```python
from build123d import *

# Parameters (mm, degrees)
F1_DEPTH = 25.4
F3_D     = 6.35
F3_DEPTH = 0.0254
F3_TIP   = 1.9077324654
F5_D     = 6.35


with BuildPart() as f1:
    # F0 (on Right) → F1 (new body)
    with BuildSketch(Plane.YZ):
        Polygon((19.0030846266, 19.1524188638), (12.6530846266, 19.1524188638), (12.6530846266, -6.2475811362), (-25.4469153734, -6.2475811362), (-25.4469153734, -12.5975811362), (19.0030846266, -12.5975811362), align=None)
    extrude(amount=F1_DEPTH)

    # F3
    with Locations(Plane(origin=(0, 19.0030846266, 0), x_dir=(-1, 0, 0), z_dir=(0, 1, 0))):
        with Locations((-12.7, 0.1024188638)):
            Hole(F3_D / 2, depth=F3_DEPTH)
            with Locations((0, 0, -(F3_DEPTH + F3_TIP / 2))):  # 118° drill point
                Cone(0, F3_D / 2, F3_TIP, mode=Mode.SUBTRACT)

    # F5 (through all)
    with Locations(Plane.XY.offset(-6.2475811362)):
        with Locations((12.7, -5.1269153734)):
            Hole(F5_D / 2)


solid = f1.part
```
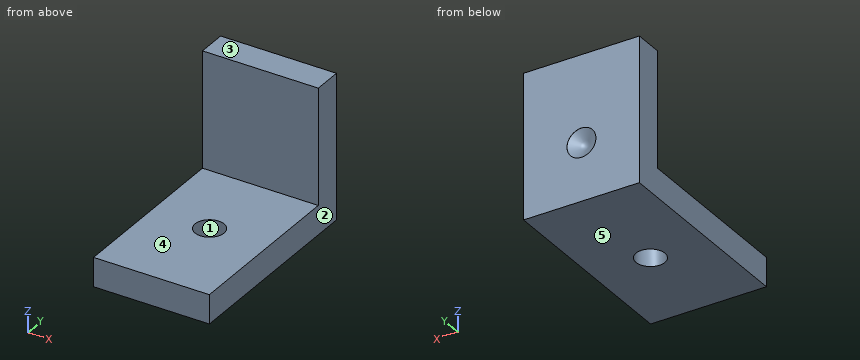
Geometry check sheet. Reference: the model listing, model coordinates, mm. Face numbers are marked on the shaded views. A direction names the side the tool comes from. Give positions to 0.01 mm unless a question says otherwise; leave off trailing zeros. Order: outer loops, then holes, each group sorted by start corner. A loop starts at its lowest first (then second) coordinate and runs counter-clockwise, first axis right, second up. Notation, with made-up numbers: (44, 48) -> (103, 48) arc R18 cw to (103, 77) -> close; hole circle Ø7 at (84, 48). An arc over 180 degrees is marked (long way). Write each question's results on one line, items separated by ' | '. Start each with the question number.
(1) Gauge pin test, flat ends, axial feed: P1, Ø12.5, axis at x = 16, z = 8.5, coming from the -Y side; P2, Ø8, axis at x = 19, y = -21, coming from the +Z side. Record the tip position at first contact, or that the pin passes through.
(2) Mould release check, pull along X, two halves, no side actions. Record for the marked faces 1, 2 and 3: pulls with the +X half, pulls with the -X half, needs draft (parallel to the pull), parting line crosses it, or undercut.
(3) Sectioned sample at A-A (z = 13.5). Enter the section's corners in (x, y).
(4) Scan lines: line 1 (Y direction, x = 12.7, z = -8); line 2 (Y direction, x = 1, z = 11); line 3 (Z direction, x = 16.25, y = -6.5). Record each from-to range of solid material in increasing order.
(5) Sectioned sample at C-C (y = -10). Enter the section's corners in (x, z).
(6) Sectioned sample at B-B (x = 17.25). Enter the section's corners in (y, z).
(7) Access from +Z, -Z, +X, -X, +Y, -Y to the whole of each face (thin tool, end or side, straight path). Record for the marked faces 4 and 5.
Answer below:
1) P1: y = 12.65 | P2: z = -6.25
2) face 1: undercut | face 2: pulls with the +X half | face 3: needs draft
3) outline: (0, 12.65) -> (25.4, 12.65) -> (25.4, 19) -> (0, 19) -> close
4) line 1: -25.45 to -8.3, -1.95 to 19 | line 2: 12.65 to 19 | line 3: -12.6 to -6.25
5) outline: (0, -12.6) -> (25.4, -12.6) -> (25.4, -6.25) -> (0, -6.25) -> close
6) outline: (-25.45, -12.6) -> (19, -12.6) -> (19, 19.15) -> (12.65, 19.15) -> (12.65, -6.25) -> (-25.45, -6.25) -> close
7) face 4: +Z, +X, -X, -Y | face 5: -Z, +X, -X, +Y, -Y
